```python
from build123d import *

# Parameters (mm, degrees)
EXTRUDE_1_DEPTH     = 2.5
SKETCH_2_W          = 15.8
SKETCH_2_H          = 6.5
EXTRUDE_2_DEPTH     = 1
FILLET_1_R          = 0.5
CHAMFER_1_SIZE      = 0.5
CUT_EXTRUDE_1_DEPTH = 12.419391402


with BuildPart() as part:
    # 草图1 → 凸台-拉伸1 (new body)
    with BuildSketch(Plane.XY):
        with BuildLine():
            Line((-9.05, -1.25), (-9.05, -3.45))
            ThreePointArc((-9.05, -3.45), (-8.713172798, -4.263172798), (-7.9, -4.6))
            Line((-7.9, -4.6), (7.9, -4.6))
            ThreePointArc((7.9, -4.6), (8.713172798, -4.263172798), (9.05, -3.45))
            Line((9.05, -3.45), (9.05, -1.25))
            ThreePointArc((9.05, -1.25), (8.713172798, -0.436827202), (7.9, -0.1))
            Line((7.9, -0.1), (-7.9, -0.1))
            ThreePointArc((-7.9, -0.1), (-8.713172798, -0.436827202), (-9.05, -1.25))
        make_face()
    extrude(amount=-EXTRUDE_1_DEPTH)

    # 草图2 → 凸台-拉伸2 (add)
    with BuildSketch(Plane(origin=(0, 0, -2.5), x_dir=(-1, 0, 0), z_dir=(0, 0, -1))):
        with Locations((0, -2.35)):
            Rectangle(SKETCH_2_W, SKETCH_2_H)
    extrude(amount=-EXTRUDE_2_DEPTH)

    # 圆角1
    fillet_1_edges = [part.edges().sort_by_distance(p)[0] for p in [
        (-7.9, 0.9, -2),
        (-7.9, -5.6, -2),
        (7.9, -5.6, -2),
        (7.9, 0.9, -2),
    ]]
    fillet(fillet_1_edges, radius=FILLET_1_R)

    # 倒角1
    chamfer_1_edges = [part.edges().sort_by_distance(p)[0] for p in [
        (-9.05, -2.35, 0),
        (-8.713172798, -0.436827202, 0),
        (0, -0.1, 0),
        (8.713172798, -0.436827202, 0),
        (9.05, -2.35, 0),
        (8.713172798, -4.263172798, 0),
        (0, -4.6, 0),
        (-8.713172798, -4.263172798, 0),
    ]]
    chamfer(chamfer_1_edges, length=CHAMFER_1_SIZE)

    # 草图3 → 切除-拉伸1 (cut, through all)
    with BuildSketch(Plane(origin=(0, 0.9, 0), x_dir=(1, 0, 0), z_dir=(0, 1, 0))):
        Polygon((8.475, 2.5), (9.05, 1.925), (9.05, 2.5), align=None)
        Polygon((-9.05, 1.925), (-9.05, 2.5), (-8.475, 2.5), align=None)
    extrude(amount=-CUT_EXTRUDE_1_DEPTH, mode=Mode.SUBTRACT)


solid = part.part
```
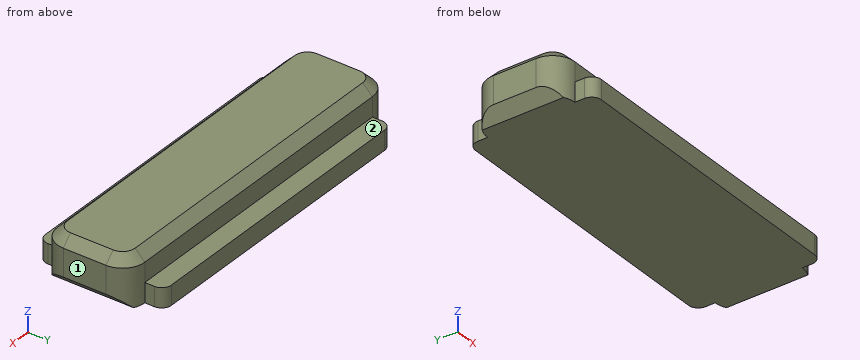
Geometry: final body of the model. Coordinates: model frame, mm. Face numbers are marked on the shaded views. A direction names the side the tool comes from. Round coordinates to 2 decimals unless told otherwise and drop trailing zeros. Order: outer loops, then holes, each group sorted by start corner. A loop starts at its lowest first (then second) coordinate and runs counter-clockwise, first axis right, second up. Notation, with made-up numbers: (-16.75, 19.25) - (37.25, 19.25) arc R26 ccw to (37.25, 36.25) - close; hole circle Ø3 at (73.5, 46.25). An arc over 180 degrees is marked (long way). Write item = value, one per line. Start each with the question number.
Q1. Cut plane A-A on z = -1.75. Return the cut outline in (x, y).
Q2. Access query for the marked faces 1 and 2. Directions: +Z, -Z, +X, -X, +Y, -Y. A direction counts if a zero-diameter tool reaches every point of the face in a straight line with its end or side. Return the directions, or none.
Q3. Cut plane C-C on z = -0.7. Return the cut outline in (x, y), and give its area (3 significant figures).
Q4. Cut plane B-B on x = -0.75. Return the cut outline in (y, z).
Q5. Ray query, line 1 (Z direction, x = 2.75, y = -0.5); line 2 (Y direction, x = 1.5, z = -1.3); line 3 (X direction, y = -4.75, z = -1.9). Return the intervals inside material, ascending. Write a range as from..to.
Q6. Pin query (flat end, axial travel): pin 1 (1.1 mm diameter, centred on x = -3.5, y = 0.5, fed in from +Z); pin 2 (0.5 mm diameter, centred on x = 2.5, z = -1, fed in from +Y); pin 3 (0.8 mm diameter, centred on x = -3, z = -1, fed in from -Y). Return the tip coordinate at first contact, or that it passes through.
Outcome:
q1.outline = (-9.05, -3.45) arc R1.15 ccw to (-7.9, -4.6) - (-7.9, -5.1) arc R0.5 ccw to (-7.4, -5.6) - (7.4, -5.6) arc R0.5 ccw to (7.9, -5.1) - (7.9, -4.6) arc R1.15 ccw to (9.05, -3.45) - (9.05, -1.25) arc R1.15 ccw to (7.9, -0.1) - (7.9, 0.4) arc R0.5 ccw to (7.4, 0.9) - (-7.4, 0.9) arc R0.5 ccw to (-7.9, 0.4) - (-7.9, -0.1) arc R1.15 ccw to (-9.05, -1.25) - close
q2.face_1 = +Z, -Z, +X, +Y, -Y
q2.face_2 = +Z, +X, -X, +Y
q3.outline = (-9.05, -3.45) arc R1.15 ccw to (-7.9, -4.6) - (7.9, -4.6) arc R1.15 ccw to (9.05, -3.45) - (9.05, -1.25) arc R1.15 ccw to (7.9, -0.1) - (-7.9, -0.1) arc R1.15 ccw to (-9.05, -1.25) - close
q3.area = 80.3 mm^2
q4.outline = (-5.6, -2.5) - (0.9, -2.5) - (0.9, -1.5) - (-0.1, -1.5) - (-0.1, -0.5) - (-0.6, 0) - (-4.1, 0) - (-4.6, -0.5) - (-4.6, -1.5) - (-5.6, -1.5) - close
q5.line_1 = -2.5..-0.1
q5.line_2 = -4.6..-0.1
q5.line_3 = -7.9..7.9
q6.pin_1 = -1.5
q6.pin_2 = -0.1
q6.pin_3 = -4.6
